Print and shaded views of the part. All mm, measured from the part's lowest x, y and z. Coordinates: 2 decimals unless noted, no trailing zeros. Order: outer loops, then holes, each group sorted by start corner. A loop starts at its lowest first (then second) coordinate and runs counter-clockwise, first axis right, second up.
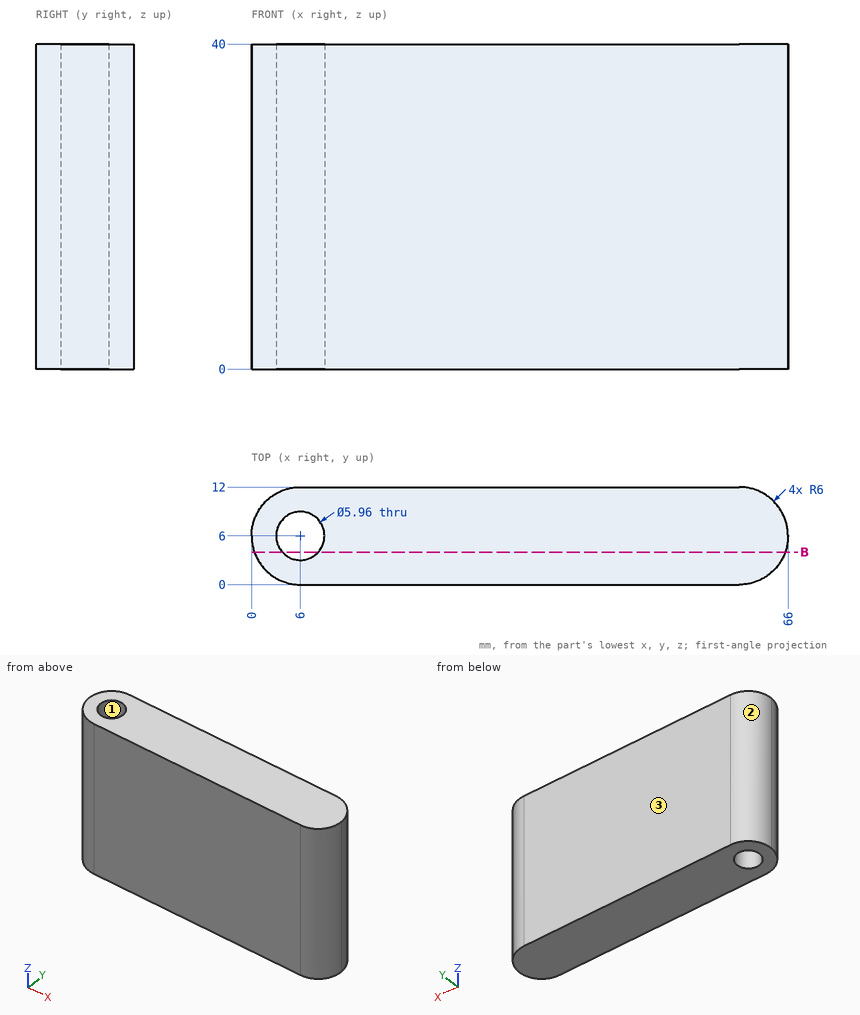
Q1. Probe line 1 (Y direction, x = 6, z = 20.5); line 2 (X direction, y = 5.75, z = 38) (1 decimal); line 3 (X direction, y = 7, z = 17.5). List the from-to ranges inside material, lowest first.
Established:
line 1: y = 0 to 3.02, 8.98 to 12
line 2: x = 0 to 3, 9 to 66
line 3: x = 0.08 to 3.19, 8.81 to 65.92
Q2. Mould opens along X. For the marked faces 1, 2 and 3 say: pulls with the +X half, pulls with the -X half, needs draft (parallel to the pull), parting line crosses it, or undercut.
Established:
face 1: undercut
face 2: pulls with the -X half
face 3: needs draft
Q3. Cut at B-B, the plane y = 4. List the corners of the cut face in (x, z).
Established:
outline: (0.34, 0) - (3.79, 0) - (3.79, 40) - (0.34, 40) - close; (8.21, 0) - (65.66, 0) - (65.66, 40) - (8.21, 40) - close
Q4. Drop a flat-ended pin along its axis: P1, Ø1.5, axis at y = 8.5, z = 30, coming from the -X side. Give the stop position or say it passes through.
Established:
P1: stops at x = 0.26
